Input: part model. Units: mm. Frame: model coordinates. A direction names the side the tool comes from. Coordinates: 2 decimals unless noted, no trailing zeros. Loops run counter-clockwise (first coordinate to the right, second up) from the corner with the lowest first, then second, coordinate; pieces in that order, holes last. Notation, with made-up numbers: (38, 73.5) - (57, 73.5) arc R19 ccw to (57, 95.5) - close; hole circle Ø6 at (20.5, 88.5). An arc over 180 degrees is marked (long way). Write item = value, one per line. Start each with the question number.
from build123d import *

# Parameters (mm, degrees)
SKETCH_1_W          = 15
SKETCH_1_H          = 15
SKETCH_1_W_2        = 12
SKETCH_1_H_2        = 12
EXTRUDE_1_DEPTH     = 666
SKETCH_2_R          = 2.15
CUT_EXTRUDE_1_DEPTH = 667.211115188
SKETCH_3_R          = 2.15
CUT_EXTRUDE_2_DEPTH = 667.211115188


with BuildPart() as part:
    # ｽｹｯﾁ1 → 押し出し-薄板1 (new body)
    with BuildSketch(Plane.XY):
        Rectangle(SKETCH_1_W, SKETCH_1_H)
        Rectangle(SKETCH_1_W_2, SKETCH_1_H_2, mode=Mode.SUBTRACT)
    extrude(amount=EXTRUDE_1_DEPTH)

    # ｽｹｯﾁ2 → ｶｯﾄ - 押し出し1 (cut, through all)
    with BuildSketch(Plane(origin=(7.5, 0, 0), x_dir=(0, 0, -1), z_dir=(1, 0, 0))):
        with Locations(Location((-5, -2.5, 0), (0, 0, 90))):
            Circle(SKETCH_2_R)
        with Locations(Location((-661, -2.5, 0), (0, 0, 90))):
            Circle(SKETCH_2_R)
        with Locations(Location((-25, -2.5, 0), (0, 0, 90))):
            Circle(SKETCH_2_R)
        with Locations(Location((-641, -2.5, 0), (0, 0, 90))):
            Circle(SKETCH_2_R)
    extrude(amount=-CUT_EXTRUDE_1_DEPTH, mode=Mode.SUBTRACT)

    # ｽｹｯﾁ3 → ｶｯﾄ - 押し出し2 (cut, through all)
    with BuildSketch(Plane(origin=(0, 7.5, 0), x_dir=(1, 0, 0), z_dir=(0, 1, 0))):
        with Locations(Location((-2.5, -228, 0), (0, 0, 270))):
            Circle(SKETCH_3_R)
        with Locations(Location((-2.5, -438, 0), (0, 0, 270))):
            Circle(SKETCH_3_R)
        with Locations(Location((-2.5, -183, 0), (0, 0, 270))):
            Circle(SKETCH_3_R)
        with Locations(Location((-2.5, -483, 0), (0, 0, 270))):
            Circle(SKETCH_3_R)
        with Locations(Location((0, -373, 0), (0, 0, 270))):
            Circle(SKETCH_3_R)
        with Locations(Location((0, -293, 0), (0, 0, 270))):
            Circle(SKETCH_3_R)
    extrude(amount=-CUT_EXTRUDE_2_DEPTH, mode=Mode.SUBTRACT)


solid = part.part
Item 1: Access query for faces 5 (the flat face through (7.5, 0, 328)), 6 (the flat face through (-6, 0, 328)). Directions: +Z, -Z, +X, -X, +Y, -Y. A direction counts if a zero-diameter tool reaches every point of the face in a straight line with its end or side. Return the directions, or none.
Item 2: Pull-direction query (Y, two-part tool) for faces 1 (the flat face through (0, 7.5, 328)), 2 (the flat face through (6, 0, 328)), 3 (the flat face through (0, 6, 328)), 4 (the flat face through (-7, 0, 666)); classes: pulls with the +Y half, pulls with the -Y half, needs draft (parallel to the pull), parting line crosses it, or undercut.
Item 3: Cut plane A-A on z = 145.5. Return loops of the section in (x, y), plus the area to 3 significant figures.
Item 4: Ray query, line 1 (Z direction, x = -6.4, y = -2.5); line 2 (Y direction, x = -1.75, z = 125.5). Return the intervals inside material, ascending.
Item 5: Pin query (flat end, axial travel): pin 1 (4 mm diameter, centred on x = 0, z = 293, fed in from +Y). Return the tip coordinate at first contact, or that it passes through.
Recorded:
q1.face_5 = +Z, -Z, +X, +Y, -Y
q1.face_6 = +Z, -Z
q2.face_1 = pulls with the +Y half
q2.face_2 = undercut
q2.face_3 = undercut
q2.face_4 = needs draft
q3.outline = (-7.5, -7.5) - (7.5, -7.5) - (7.5, 7.5) - (-7.5, 7.5) - close; hole (-6, -6) - (6, -6) - (6, 6) - (-6, 6) - close
q3.area = 81.0 mm²
q4.line_1 = 0 to 2.85, 7.15 to 22.85, 27.15 to 638.85, 643.15 to 658.85, 663.15 to 666
q4.line_2 = -7.5 to -6, 6 to 7.5
q5.pin_1 = through
